```python
from build123d import *

# Parameters (mm, degrees)
BOSS_EXTRUDE1_START = 56
SKETCH1_W           = 22
SKETCH1_H           = 30
BOSS_EXTRUDE1_DEPTH = 10
BOSS_EXTRUDE2_START = 58
SKETCH2_W           = 14
SKETCH2_H           = 8
BOSS_EXTRUDE2_DEPTH = 6


with BuildPart() as part:
    # Sketch1 → Boss-Extrude1 (new body)
    with BuildSketch(Plane.XY.offset(BOSS_EXTRUDE1_START)):
        with Locations((41, 173)):
            Rectangle(SKETCH1_W, SKETCH1_H)
    extrude(amount=BOSS_EXTRUDE1_DEPTH)

    # Sketch2 → Boss-Extrude2 (add)
    with BuildSketch(Plane.XY.offset(BOSS_EXTRUDE2_START)):
        with Locations((41, 192)):
            Rectangle(SKETCH2_W, SKETCH2_H)
    extrude(amount=BOSS_EXTRUDE2_DEPTH)


solid = part.part
```
Input: part model. Units: mm. Frame: model coordinates. A direction names the side the tool comes from. Give positions to 0.01 mm unless a question says otherwise; leave off trailing zeros. Write each loop counter-clockwise with the first axis right and the second up, starting at its lowest first coordinate (ties: lowest second). Pieces come first, ordered by that corner, then holes. Notation, with made-up numbers: (63.5, -5) - (86.5, -5) arc R9 ccw to (86.5, 5) - close; hole circle Ø4 at (73, -9.5). An arc over 180 degrees is marked (long way). Write item = value, one per line. Start each with the question number.
1) Cut plane C-C (z = 57.5). Return loops of the section in (x, y).
2) Material intervals for L1, parallel to Y at x = 32.25, z = 60.25; L2, parallel to X at y = 189, z = 59.5, sorted ascending. Write a range as [from, to].
3) Reachability of faces 1 (the face through (41, 192, 58)), 2 (the face through (41, 192, 64)), 3 (the face through (34, 192, 61)), 4 (the face through (48, 192, 61)) from +Z, -Z, +X, -X, +Y, -Y: full face, straight path, thin tool, end or side. Return the list, or none.
4) Cut plane A-A (z = 61.5). Return loops of the section in (x, y).
5) Pin query (flat end, axial travel): pin 1 (5 mm diameter, centred on y = 191.5, z = 62, fed in from -X); pin 2 (6.5 mm diameter, centred on x = 44, y = 193, fed in from -Z). Return the tip coordinate at first contact, or that it passes through.
6) Cut plane B-B (x = 37.25). Return loops of the section in (y, z), and give its area (3 significant figures).
Answers follow:
q1.outline = (30, 158) - (52, 158) - (52, 188) - (30, 188) - close
q2.L1 = [158, 188]
q2.L2 = [34, 48]
q3.face_1 = -Z, +X, -X, +Y
q3.face_2 = +Z, +X, -X, +Y
q3.face_3 = +Z, -Z, -X, +Y
q3.face_4 = +Z, -Z, +X, +Y
q4.outline = (30, 158) - (52, 158) - (52, 188) - (48, 188) - (48, 196) - (34, 196) - (34, 188) - (30, 188) - close
q5.pin_1 = 34
q5.pin_2 = 58
q6.outline = (158, 56) - (188, 56) - (188, 58) - (196, 58) - (196, 64) - (188, 64) - (188, 66) - (158, 66) - close
q6.area = 348 mm^2
